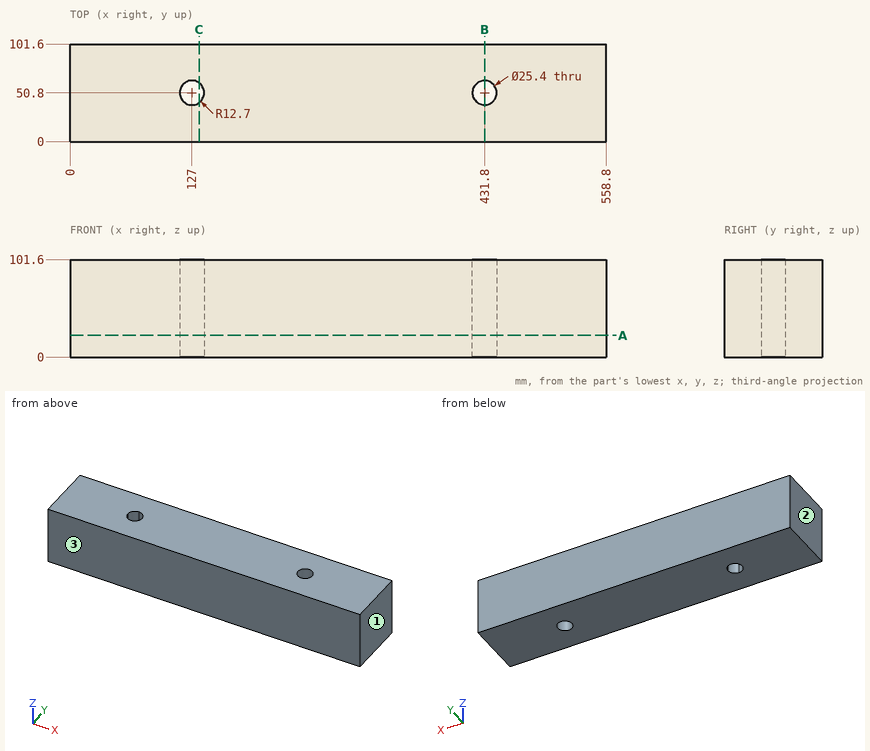
Can you work these out from the drawing? Everything is in mm from the part's minimum corner. Coordinates: 2 decimals unless noted, no trailing zeros. Write each loop counter-clockwise with the first axis right and the second up, starting at its lowest first coordinate (ties: lowest second). Pieces come first, ordered by that corner, then holes. Notation, with made-up numbers: (-6, 32.25) - (3, 32.25) arc R8 ccw to (3, 40.25) - close; hole circle Ø5 at (53.25, 46.5). An arc over 180 degrees is marked (long way). Use a Markdown table: item, result.
Q1. I'm going to push a flat-ended pin straight in: pin 1 Ø5 at (y, z) = (72, 34) entering from -X. Where does the tip first touch, or does it pass through?
Geometry check:
| item | result |
|---|---|
| pin 1 | stops at x = 0 |
Q2. Imagine slicing it at A-A (z = 22.5). List the corners of the cut face in (x, y) for me.
Geometry check:
| item | result |
|---|---|
| outline | (0, 0) - (558.8, 0) - (558.8, 101.6) - (0, 101.6) - close; hole circle Ø25.4 at (127, 50.8); hole circle Ø25.4 at (431.8, 50.8) |
Q3. Thinking about a two-plate mould opening in X: for the marked faces 1, 2 and 3, which applies, +X half, -X half, draft (parallel to the pull), parting line (faces both ways), or undercut?
Geometry check:
| item | result |
|---|---|
| face 1 | +X half |
| face 2 | -X half |
| face 3 | draft |
Q4. Imagine slicing it at C-C (x = 134.5). List the corners of the cut face in (y, z) for me.
Geometry check:
| item | result |
|---|---|
| outline | (0, 0) - (40.55, 0) - (40.55, 101.6) - (0, 101.6) - close; (61.05, 0) - (101.6, 0) - (101.6, 101.6) - (61.05, 101.6) - close |
Q5. Imagine slicing it at B-B (x = 431.8). List the corners of the cut face in (y, z) for me, and give its area (3 significant figures).
Geometry check:
| item | result |
|---|---|
| outline | (0, 0) - (38.1, 0) - (38.1, 101.6) - (0, 101.6) - close; (63.5, 0) - (101.6, 0) - (101.6, 101.6) - (63.5, 101.6) - close |
| area | 7,740 mm2 |
Q6. Please list where these lines run through material, in increasing order: L1, parallel to X at y = 50, z = 35; L2, parallel to Y at x = 431.8, z = 41.5; L3, parallel to X at y = 42, z = 73.
Geometry check:
| item | result |
|---|---|
| L1 | x = 0 to 114.33, 139.67 to 419.13, 444.47 to 558.8 |
| L2 | y = 0 to 38.1, 63.5 to 101.6 |
| L3 | x = 0 to 117.84, 136.16 to 422.64, 440.96 to 558.8 |
